Build history of the part. All positions in model axes, mm. Face numbers are marked on the shaded views. Round coordinates to 2 decimals unless told otherwise and drop trailing zeros. Write each loop counter-clockwise with the first axis right and the second up, starting at its lowest first coordinate (ties: lowest second). Pieces come first, ordered by that corner, then holes. Notation, with made-up numbers: (76.25, 18.25) - (98.25, 18.25) arc R27 ccw to (98.25, 40.25) - close; hole circle Ø5 at (79, 35). An arc over 180 degrees is marked (long way). Answer as a JSON object with one key per item and string values. Group by question number.
Item 1: Probe line 1 (X direction, y = -6.5, z = 12); line 2 (X direction, y = 0, z = 12.25); line 3 (Y direction, x = 1.5, z = 13). List the from-to ranges inside material, lowest first. Write a range as from..to.
Item 2: Two-plate mould, pull along Y, no slides. Class the marked faces 1, 2 and 3: +Y half, -Y half, draft (parallel to the pull), parting line (faces both ways), or undercut.
Item 3: Flat gauge pins, fed straight in: pin 1 (5 mm diameter, centred on x = -76, z = 4.5, fed in from -Y); pin 2 (9 mm diameter, centred on x = -84.5, z = 7, fed in from -Y); pin 3 (6.5 mm diameter, centred on x = -23.5, z = 5.5, fed in from +Y); pin 4 (6 mm diameter, centred on x = 3, y = 9.5, fed in from +Z). Where does each tip first touch, or does it go through?
Item 4: Slice it at B-B, the plane z = 5.5. List the corners of the cut face in (x, y), then the cut area to 3 significant figures.
Item 5: Slice it at A-A, the plane x = -9. List the corners of the cut face in (y, z).
from build123d import *

# Parameters (mm, degrees)
F0_R     = 17.5
F0_W     = 10
F0_H     = 30
F0_W_2   = 8
F0_H_2   = 15
F1_DEPTH = 15
F2_R     = 2


with BuildPart() as f1:
    # F0 (on Top) → F1 (new body)
    with BuildSketch(Plane.XY):
        Polygon((-109.0468041226, 32.7149193907), (-109.0468041226, 7.7149193907), (-99.0468041226, 7.7149193907), (-89.0468041226, 7.7149193907), (-81.0468041226, 7.7149193907), (-71.0468041226, 7.7149193907), (-57.0468041226, 7.7149193907), (45.9531958774, 7.7149193907), (45.9531958774, 32.7149193907), align=None)
        with BuildLine():
            ThreePointArc((45.9531958774, 7.7149193907), (113.6449379539, 20.2149193907), (45.9531958774, 32.7149193907))
            Line((45.9531958774, 32.7149193907), (45.9531958774, 7.7149193907))
        make_face()
        with Locations((78.6449379539, 20.2149193907)):
            Circle(F0_R, mode=Mode.SUBTRACT)
        with Locations((-104.0468041226, -7.2850806093)):
            Rectangle(F0_W, F0_H)
        with Locations((-85.0468041226, 0.2149193907)):
            Rectangle(F0_W_2, F0_H_2)
        Polygon((-57.0468041226, 7.7149193907), (-71.0468041226, 7.7149193907), (-63.7032017112, -7.2850806093), align=None)
    extrude(amount=F1_DEPTH)

    # F2
    f2_edges = [f1.edges().sort_by_distance(p)[0] for p in [
        (-109.046804, 5.214919, 15),
        (-31.546804, 32.714919, 15),
        (-99.046804, -7.285081, 15),
        (-94.046804, 7.714919, 15),
        (-85.046804, -7.285081, 15),
        (-76.046804, 7.714919, 15),
        (-67.375003, 0.214919, 15),
        (-5.546804, 7.714919, 15),
        (113.644938, 20.214919, 15),
        (61.144938, 20.214919, 15),
        (-60.375003, 0.214919, 15),
        (-81.046804, 0.214919, 15),
        (-89.046804, 0.214919, 15),
    ]]
    fillet(f2_edges, radius=F2_R)


solid = f1.part
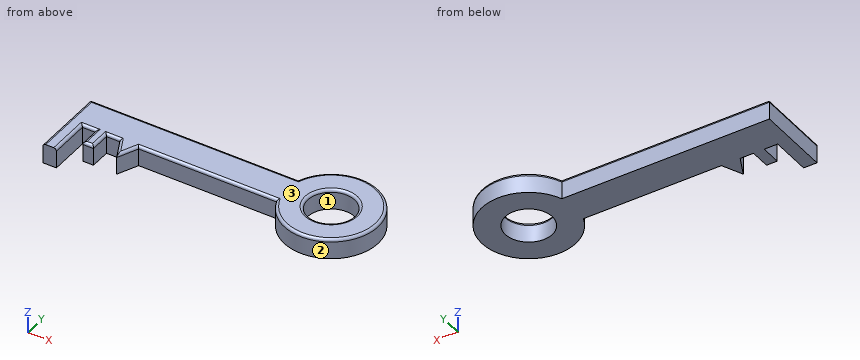
Geometry says:
{
 "1": {"line 1": "x = -109.05..-99.05, -89.05..-81.05, -64.09..-63.35, 56.03..101.26", "line 2": "x = -109.05..-99.05, -89.05..-81.05, -67.27..-60.47, 50.07..107.22", "line 3": "y = 7.71..32.71"},
 "2": {"face 1": "undercut", "face 2": "parting line", "face 3": "draft"},
 "3": {"pin 1": "stops at y = 7.71", "pin 2": "stops at y = -7.29", "pin 3": "stops at y = 32.71", "pin 4": "stops at z = 15"},
 "4": {"outline": "(-109.05, -22.29) - (-99.05, -22.29) - (-99.05, 7.71) - (-89.05, 7.71) - (-89.05, -7.29) - (-81.05, -7.29) - (-81.05, 7.71) - (-71.05, 7.71) - (-63.7, -7.29) - (-57.05, 7.71) - (45.95, 7.71) arc R35 ccw (long way) to (45.95, 32.71) - (-109.05, 32.71) - close; hole circle Ø35 at (78.64, 20.21)", "area": "7,250 mm^2"},
 "5": {"outline": "(7.71, 0) - (32.71, 0) - (32.71, 13) arc R2 ccw to (30.71, 15) - (9.71, 15) arc R2 ccw to (7.71, 13) - close"}
}
